```python
from build123d import *

# Parameters (mm, degrees)
SKETCH3_R           = 1.5
BOSS_EXTRUDE1_DEPTH = 5.13


with BuildPart() as part:
    # Sketch3 → Boss-Extrude1 (new body)
    with BuildSketch(Plane(origin=(0, 0, 0), x_dir=(1, 0, 0), z_dir=(0, 1, 0))):
        with BuildLine():
            Line((-15.990914087, -2.635364826), (-15.990914087, -9.436864826))
            Line((-15.990914087, -9.436864826), (-21.120914087, -9.436864826))
            Line((-21.120914087, -9.436864826), (-21.120914087, -26.036864826))
            Line((-21.120914087, -26.036864826), (-15.990914087, -26.036864826))
            Line((-15.990914087, -26.036864826), (-15.990914087, -48.316864826))
            Line((-15.990914087, -48.316864826), (12.009085913, -48.316864826))
            ThreePointArc((12.009085913, -48.316864826), (12.716192694, -48.023971608), (13.009085913, -47.316864826))
            Line((13.009085913, -47.316864826), (13.009085913, 45.043135174))
            ThreePointArc((13.009085913, 45.043135174), (12.716192694, 45.750241955), (12.009085913, 46.043135174))
            Line((12.009085913, 46.043135174), (-15.990914087, 46.043135174))
            Line((-15.990914087, 46.043135174), (-15.990914087, 23.763135174))
            Line((-15.990914087, 23.763135174), (-21.120914087, 23.763135174))
            Line((-21.120914087, 23.763135174), (-21.120914087, 7.163135174))
            Line((-21.120914087, 7.163135174), (-15.990914087, 7.163135174))
            Line((-15.990914087, 7.163135174), (-15.990914087, 0.361635174))
            Line((-15.990914087, 0.361635174), (-11.995914087, 0.361635174))
            Line((-11.995914087, 0.361635174), (-11.995914087, 1.720635174))
            Line((-11.995914087, 1.720635174), (-9.828914087, 1.720635174))
            Line((-9.828914087, 1.720635174), (-9.828914087, 0.361635174))
            Line((-9.828914087, 0.361635174), (-3.621914087, 0.361635174))
            Line((-3.621914087, 0.361635174), (-3.621914087, -2.635364826))
            Line((-3.621914087, -2.635364826), (-9.828914087, -2.635364826))
            Line((-9.828914087, -2.635364826), (-9.828914087, -3.994364826))
            Line((-9.828914087, -3.994364826), (-11.995914087, -3.994364826))
            Line((-11.995914087, -3.994364826), (-11.995914087, -2.635364826))
            Line((-11.995914087, -2.635364826), (-15.990914087, -2.635364826))
        make_face()
        with Locations((-1.490914087, -38.750864826)):
            Circle(SKETCH3_R, mode=Mode.SUBTRACT)
        with Locations((-1.490914087, 36.477135174)):
            Circle(SKETCH3_R, mode=Mode.SUBTRACT)
    extrude(amount=BOSS_EXTRUDE1_DEPTH)


solid = part.part
```
Design review of the part built by this model. Coordinates are the model's own, in mm. A direction names the side the tool comes from. Coordinates: 2 decimals unless noted, no trailing zeros. Write each loop counter-clockwise with the first axis right and the second up, starting at its lowest first coordinate (ties: lowest second). Pieces come first, ordered by that corner, then holes.
1) Add section B-B (y = 4.25). Write out the cut boundary in (x, z).
2) Insertion check: pin 1 (0.7 mm diameter, centred on y = 1.5, z = -1, fed in from -X); pin 2 (2.5 mm diameter, centred on x = -17.5, y = 3, fed in from +Z); pin 3 (2.5 mm diameter, centred on x = -1.49, z = -36.48, fed in from -Y). Each pin has a flat end and moves straight along its axis. Give the tip position at first contact, or say it passes through.
3) Add section C-C (z = 6.5). Write out the cut boundary in (x, y).
4) To check wall thickness, follow L1, parallel to Z at x = -1.5, y = 3.7; L2, parallel to Z at x = -5, y = 4.2; L3, parallel to Z at x = -20, y = 0.55. State the ranges of each line that lie inside material, in increasing order.
5) Machinability: for faces 4 (the flat face through (-14, 3, -0.362)), 5 (the flat face through (-11, 3, 3.994)), 6 (the flat face through (-21.121, 3, -16)), 7 (the flat face through (-15.991, 3, -35)), 8 (the flat face through (-1, 0, 0)), which of the approach directions +Z, -Z, +X, -X, +Y, -Y give a long, thin tool a straight path to every point of the face, cutting with its end or side? Answer none if there is none.
6) Mouldability with a two-part tool opening along Z and no side actions: class faces 1 (the flat face through (-19, 3, 26.037)), 2 (the flat face through (13.009, 3, 2)), 3 (the flat face through (-3.622, 3, 1)) as +Z half, -Z half, draft (parallel to the pull), parting line (faces both ways), or undercut.
7) Add section A-A (x = -8). Write out the cut boundary in (y, z).
Check result:
1. outline: (-21.12, -23.76) - (-15.99, -23.76) - (-15.99, -46.04) - (12.01, -46.04) arc R1 ccw to (13.01, -45.04) - (13.01, 47.32) arc R1 ccw to (12.01, 48.32) - (-15.99, 48.32) - (-15.99, 26.04) - (-21.12, 26.04) - (-21.12, 9.44) - (-15.99, 9.44) - (-15.99, 2.64) - (-12, 2.64) - (-12, 3.99) - (-9.83, 3.99) - (-9.83, 2.64) - (-3.62, 2.64) - (-3.62, -0.36) - (-9.83, -0.36) - (-9.83, -1.72) - (-12, -1.72) - (-12, -0.36) - (-15.99, -0.36) - (-15.99, -7.16) - (-21.12, -7.16) - close; hole circle Ø3 at (-1.49, -36.48); hole circle Ø3 at (-1.49, 38.75)
2. pin 1: stops at x = -15.99
2. pin 2: stops at z = 26.04
2. pin 3: passes through
3. outline: (-15.99, 0) - (13.01, 0) - (13.01, 5.13) - (-15.99, 5.13) - close
4. L1: z = -46.04 to -37.98, -34.98 to 37.25, 40.25 to 48.32
4. L2: z = -46.04 to -0.36, 2.64 to 48.32
4. L3: z = -23.76 to -7.16, 9.44 to 26.04
5. face 4: -X, +Y, -Y
5. face 5: +Y, -Y
5. face 6: +Z, -Z, -X, +Y, -Y
5. face 7: -Z, -X, +Y, -Y
5. face 8: +Z, -Z, +X, -X, -Y
6. face 1: +Z half
6. face 2: draft
6. face 3: undercut
7. outline: (0, -46.04) - (5.13, -46.04) - (5.13, -0.36) - (0, -0.36) - close; (0, 2.64) - (5.13, 2.64) - (5.13, 48.32) - (0, 48.32) - close
